Source: CAD feature listing. Evaluate the final solid. Frame: model axes, mm. A direction names the side the tool comes from. Coordinates: 2 decimals unless noted, no trailing zeros. Loops run counter-clockwise (first coordinate to the right, second up) from the corner with the lowest first, then second, coordinate; pieces in that order, holes last. Notation, with made-up numbers: (58, 71) -> (62, 71) arc R29 cw to (62, 91) -> close; hole circle Ø6 at (-3.75, 23). An arc over 180 degrees is marked (long way). Answer as CSV lines item,"result".
from build123d import *

# Parameters (mm, degrees)
SKETCH1_W           = 42
SKETCH1_H           = 82
BOSS_EXTRUDE1_DEPTH = 23
SKETCH2_W           = 18
SKETCH2_H           = 18
BOSS_EXTRUDE2_DEPTH = 20
SKETCH3_R           = 3.2
CUT_EXTRUDE1_DEPTH  = 21
SKETCH4_R           = 18.8
BOSS_EXTRUDE3_DEPTH = 267
SKETCH5_R           = 20
BOSS_EXTRUDE4_DEPTH = 126
SKETCH6_R           = 10
CUT_EXTRUDE2_DEPTH  = 20
SKETCH7_R           = 14
CUT_EXTRUDE5_DEPTH  = 247


with BuildPart() as part:
    # Sketch1 → Boss-Extrude1 (new body)
    with BuildSketch(Plane.XY):
        Rectangle(SKETCH1_W, SKETCH1_H)
    extrude(amount=BOSS_EXTRUDE1_DEPTH)

    # Sketch2 → Boss-Extrude2 (add)
    with BuildSketch(Plane.XY.offset(23)):
        with Locations((0, -17)):
            Rectangle(SKETCH2_W, SKETCH2_H)
    extrude(amount=BOSS_EXTRUDE2_DEPTH)

    # Sketch3 → Cut-Extrude1 (cut)
    with BuildSketch(Plane(origin=(9, 0, 0), x_dir=(0, 0, -1), z_dir=(1, 0, 0))):
        with Locations(Location((-35, -17, 0), (0, 0, 90))):
            Circle(SKETCH3_R)
    extrude(amount=-CUT_EXTRUDE1_DEPTH, mode=Mode.SUBTRACT)

    # Sketch4 → Boss-Extrude3 (add)
    with BuildSketch(Plane(origin=(0, 0, 0), x_dir=(-1, 0, 0), z_dir=(0, 0, -1))):
        with Locations((0, -19.778983504)):
            Circle(SKETCH4_R)
    extrude(amount=BOSS_EXTRUDE3_DEPTH)

    # Sketch5 → Boss-Extrude4 (add)
    with BuildSketch(Plane(origin=(0, 0, 0), x_dir=(-1, 0, 0), z_dir=(0, 0, -1))):
        with Locations((0, 20.401687075)):
            Circle(SKETCH5_R)
    extrude(amount=BOSS_EXTRUDE4_DEPTH)

    # Sketch6 → Cut-Extrude2 (cut)
    with BuildSketch(Plane(origin=(0, 0, -267), x_dir=(-1, 0, 0), z_dir=(0, 0, -1))):
        with Locations((0, -19.778983504)):
            Circle(SKETCH6_R)
    extrude(amount=-CUT_EXTRUDE2_DEPTH, mode=Mode.SUBTRACT)

    # Sketch7 → Cut-Extrude5 (cut)
    with BuildSketch(Plane(origin=(0, 0, -247), x_dir=(-1, 0, 0), z_dir=(0, 0, -1))):
        with Locations((0, -19.778983504)):
            Circle(SKETCH7_R)
    extrude(amount=-CUT_EXTRUDE5_DEPTH, mode=Mode.SUBTRACT)


solid = part.part
(1) Cut plane C-C (y = -17). Return the cut outline in (x, z).
Computed values:
outline,"(-21, 0) -> (-18.59, 0) -> (-18.59, -267) -> (-9.61, -267) -> (-9.61, -247) -> (-13.72, -247) -> (-13.72, 0) -> (13.72, 0) -> (13.72, -247) -> (9.61, -247) -> (9.61, -267) -> (18.59, -267) -> (18.59, 0) -> (21, 0) -> (21, 23) -> (9, 23) -> (9, 31.8) -> (-9, 31.8) -> (-9, 23) -> (-21, 23) -> close; (-9, 38.2) -> (9, 38.2) -> (9, 43) -> (-9, 43) -> close"
(2) Pin query (flat end, axial travel): pin 1 Ø5 at (x, z) = (-10.5, -83.5) entering from -Y; pin 2 Ø3 at (x, z) = (16, -95) entering from +Y; pin 3 Ø14.5 at (x, z) = (-1, 34) entering from +Y; pin 4 Ø6 at (y, z) = (-17, 35) entering from -X. Return the tip coordinate at first contact, or that it passes through.
Computed values:
pin 1,"y = -36.79"
pin 2,"y = 34.18"
pin 3,"y = -8"
pin 4,"through"
(3) Access query for faces 1 (the flat face through (0, -8, 33)), 2 (the flat face through (-2, 0, 0)), 3 (the flat face through (0, 21, -126)), 4 (the flat face through (-9, -17, 31)). Directions: +Z, -Z, +X, -X, +Y, -Y. A direction counts if a zero-diameter tool reaches every point of the face in a straight line with its end or side. Return the directions, or none.
Computed values:
face 1,"+Z, +X, -X, +Y"
face 2,"-Z"
face 3,"-Z, +X, -X, +Y"
face 4,"+Z, -X, +Y, -Y"
(4) Cut plane B-B (x = 5). Return the cut outline in (y, z).
Computed values:
outline,"(-41, 0) -> (-37.9, 0) -> (-37.9, -267) -> (-28.44, -267) -> (-28.44, -247) -> (-32.86, -247) -> (-32.86, 0) -> (-6.7, 0) -> (-6.7, -247) -> (-11.12, -247) -> (-11.12, -267) -> (-1.66, -267) -> (-1.66, 0) -> (1.04, 0) -> (1.04, -126) -> (39.77, -126) -> (39.77, 0) -> (41, 0) -> (41, 23) -> (-8, 23) -> (-8, 43) -> (-26, 43) -> (-26, 23) -> (-41, 23) -> close; hole circle Ø6.4 at (-17, 35)"
(5) Draft query along Y for faces 5 (the flat face through (0, 41, 11)), 6 (the flat face through (0, -26, 33)), 7 (the flat face through (0, -20, 0)). Return one class per face: released by +Y, released by -Y, zero draft, split by the parting line, or undercut.
Computed values:
face 5,"released by +Y"
face 6,"released by -Y"
face 7,"undercut"
(6) Cut plane D-D (z = -98). Return the cut outline in (x, y), then the cut area to 3 significant figures.
Computed values:
outline,"circle Ø40 at (0, 20.4); circle Ø37.6 at (0, -19.78); hole circle Ø28 at (0, -19.78)"
area,"1,750 mm^2"
(7) Cut plane A-A (z = 35). Return the cut outline in (x, y).
Computed values:
outline,"(-9, -26) -> (9, -26) -> (9, -20.2) -> (-9, -20.2) -> close; (-9, -13.8) -> (9, -13.8) -> (9, -8) -> (-9, -8) -> close"
(8) Material intervals for L1, parallel to Y at x = 0.5, z = -93.5; L2, parallel to Y at x = 0, z = -259; L3, parallel to Z at x = -15, y = -35, sorted ascending. Write a range as [from, to].
Computed values:
L1,"[-38.57, -33.77], [-5.79, -0.99], [0.41, 40.4]"
L2,"[-38.58, -29.78], [-9.78, -0.98]"
L3,"[0, 23]"
